Autodesk Fusion 360 part; units mm, degrees
sketch "Esquisse1" plane through (0, 0, 0) normal (0, 0, 1) x (1, 0, 0)
  circle A0 centre (0, 0) radius 6
  dimension "d1" = 12
extrude "Extrusion1" add sketch "Esquisse1" along normal blind 104
sketch "Esquisse2" plane through (0, 0, 104) normal (0, 0, 1) x (-1, 0, 0)
  circle A0 centre (0, 0) radius 6
  circle A1 centre (0, 0) radius 2.5
  dimension "d5" = 5
extrude "Extrusion2" cut sketch "Esquisse2" against normal blind 12 contours A1
sketch "Esquisse3" plane through (0, 0, 0) normal (0, 0, -1) x (1, 0, 0)
  circle A0 centre (0, 0) radius 6
  circle A1 centre (0, 0) radius 2.5
  dimension "d8" = 5
extrude "Extrusion3" cut sketch "Esquisse3" against normal blind 12 contours A1
sketch "Esquisse4" plane through (0, 0, 104) normal (0, 0, 1) x (-1, 0, 0)
  circle A0 centre (0, 0) radius 2.5
  circle A1 centre (0, 0) radius 6
  line L0 (5, 8) -> (-5, 8)
  line L1 (-5, 8) -> (-5, -7.4606)
  line L2 (-5, -7.4606) -> (5, -7.4606)
  line L3 (5, -7.4606) -> (5, 8)
  dimension "d11" = 5
  dimension "d12" = 10
extrude "Extrusion4" cut sketch "Esquisse4" against normal blind 10 from surface at -20 contours A1 L3 | A1 L1
Here's how the part is built. I have some questions about the finished solid (model axes, mm). A direction names the side the tool comes from. Coordinates: 2 decimals unless noted, no trailing zeros. Write each loop counter-clockwise with the first axis right and the second up, starting at its lowest first coordinate (ties: lowest second). Pieces come first, ordered by that corner, then holes.
Item 1: I want a section at C-C on z = 55.5. Write out the boundary of the cut face in (x, y), and give its area (3 significant figures).
Item 2: If we mould it in two halves opening along X, with no side actions, what happens to faces 4 (the cylindrical face through (0.54, 2.44, 98.08)), 5 (the flat face through (5, 0, 79)), 6 (the flat face through (-5, 0, 79)), 7 (the flat face through (3, 0, 0))? For each: +X half, -X half, draft (parallel to the pull), parting line (faces both ways), or undercut.
Item 3: I want a section at D-D on z = 77. Write out the boundary of the cut face in (x, y).
Item 4: I want a section at B-B on y = 0. Write out the boundary of the cut face in (x, z), and give its area (3 significant figures).
Item 5: If I drill on line 1 (Y direction, x = 0, z = 95.5); line 2 (Z direction, x = 5.5, y = 0.75); line 3 (Y direction, x = -2.25, z = 7), over which ranges is the centre line in solid material (lowest first)?
Item 6: On a 3-axis mill with a long thin cutter (end or side, diameter ignored), from which of +Z, -Z, +X, -X, +Y, -Y can I reach the whole of each face in a straight line? I mean faces 1 (the flat face through (0, 0, 92)), 2 (the cylindrical face through (-6, 0, 51)), 3 (the cylindrical face through (-0.54, 2.44, 5.92)). Say none if no direction works.
Item 7: Will these pins go through, and if not, where does the flat tip stop? pin 1 (5 mm diameter, centred on x = 4, z = 64.5, fed in from -Y); pin 2 (3 mm diameter, centred on x = 0, y = 0, fed in from -Z); pin 3 (1 mm diameter, centred on y = -2.5, z = 48, fed in from -X).
Item 8: I want a section at A-A on x = 0. Write out the boundary of the cut face in (y, z), and give its area (3 significant figures).
Findings below:
1. outline: circle Ø12 at (0, 0)
1. area: 113 mm2
2. face 4: undercut
2. face 5: +X half
2. face 6: -X half
2. face 7: draft
3. outline: (-5, -3.32) arc R6 ccw to (5, -3.32) - (5, 3.32) arc R6 ccw to (-5, 3.32) - close
4. outline: (-6, 0) - (-2.5, 0) - (-2.5, 12) - (2.5, 12) - (2.5, 0) - (6, 0) - (6, 74) - (5, 74) - (5, 84) - (6, 84) - (6, 104) - (2.5, 104) - (2.5, 92) - (-2.5, 92) - (-2.5, 104) - (-6, 104) - (-6, 84) - (-5, 84) - (-5, 74) - (-6, 74) - close
4. area: 1,110 mm2
5. line 1: y = -6 to -2.5, 2.5 to 6
5. line 2: z = 0 to 74, 84 to 104
5. line 3: y = -5.56 to -1.09, 1.09 to 5.56
6. face 1: +Z
6. face 2: +Z, -Z
6. face 3: -Z
7. pin 1: stops at y = -5.81
7. pin 2: stops at z = 12
7. pin 3: stops at x = -5.66
8. outline: (-6, 0) - (-2.5, 0) - (-2.5, 12) - (2.5, 12) - (2.5, 0) - (6, 0) - (6, 104) - (2.5, 104) - (2.5, 92) - (-2.5, 92) - (-2.5, 104) - (-6, 104) - close
8. area: 1,130 mm2
